from build123d import *

# Parameters (mm, degrees)
SKETCH1_R               = 5
BOSS_EXTRUDE1_DEPTH     = 50
CUT_EXTRUDE1_DEPTH      = 51.497524692
CUT_EXTRUDE1_DEPTH_BACK = 51.497524692
SKETCH2_W               = 0.5
SKETCH2_H               = 40
CHAMFER1_SIZE           = 3


with BuildPart() as part:
    # Sketch1 → Boss-Extrude1 (new body)
    with BuildSketch(Plane.XY):
        Circle(SKETCH1_R)
    extrude(amount=BOSS_EXTRUDE1_DEPTH)

    # Sketch2 → Cut-Extrude1 (cut, two sides: drawn at the far end of the back side and taken through both)
    with BuildSketch(Plane(origin=(0, 0, 0), x_dir=(1, 0, 0), z_dir=(0, 1, 0)).offset(-CUT_EXTRUDE1_DEPTH_BACK)):
        with Locations((0, -20)):
            Rectangle(SKETCH2_W, SKETCH2_H)
        Polygon((-5, -8), (-2, -8), (-2, -10), (-5, -11.732050808), align=None)
        Polygon((2, -10), (5, -11.732050808), (5, -8), (2, -8), align=None)
        Polygon((-5, -16), (-2, -16), (-2, -18), (-5, -19.732050808), align=None)
        Polygon((2, -16), (2, -18), (5, -19.732050808), (5, -16), align=None)
        Polygon((-5, -24), (-2, -24), (-2, -26), (-5, -27.732050808), align=None)
        Polygon((2, -24), (2, -26), (5, -27.732050808), (5, -24), align=None)
        Polygon((-5, -32), (-2, -32), (-2, -34), (-5, -35.732050808), align=None)
        Polygon((2, -32), (2, -34), (5, -35.732050808), (5, -32), align=None)
    extrude(amount=CUT_EXTRUDE1_DEPTH + CUT_EXTRUDE1_DEPTH_BACK, mode=Mode.SUBTRACT)

    # Chamfer1
    chamfer1_edges = [part.edges().sort_by_distance(p)[0] for p in [
        (-5, 0, 0),
        (3.622844187, -3.446012188, 0),
    ]]
    chamfer(chamfer1_edges, length=CHAMFER1_SIZE)

    # Cut-Extrude2 cone 1 section (through the dimple's axis) → Cut-Extrude2 (revolve, cut)
    with BuildSketch(Plane(origin=(0, 0, 50), x_dir=(0, -1, 0), z_dir=(1, 0, 0))):
        Polygon((0, 0), (4.5, 0), (0, 25.520768188), align=None)
    revolve(axis=Axis((0, 0, 50), (0, 0, -1)), mode=Mode.SUBTRACT)


solid = part.part
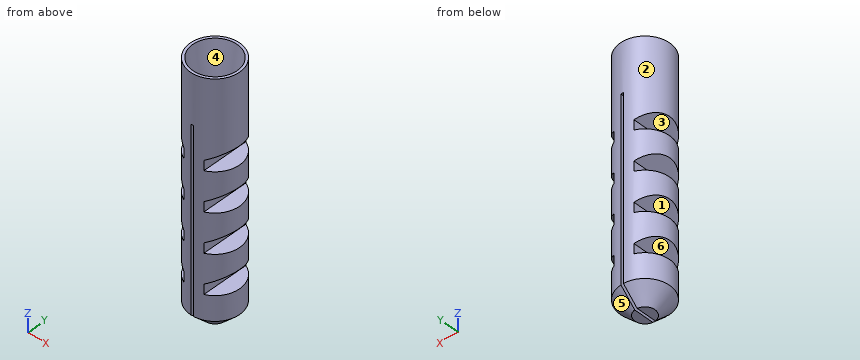
Verification items for the finished model (mm, model axes). Face numbers are marked on the shaded views. A direction names the side the tool comes from. Coordinates: 2 decimals unless noted, no trailing zeros. Order: outer loops, then holes, each group sorted by start corner. A loop starts at its lowest first (then second) coordinate and runs counter-clockwise, first axis right, second up. Notation, with made-up numbers: (63.5, -34) -> (90.5, -34) arc R28 ccw to (90.5, -2) -> close; hole circle Ø5 at (77, -24.75). An arc over 180 degrees is marked (long way). Use CSV: the item, a comma, the result in double quotes. Start each with the question number.
Q1. Draft check along Z on the marked faces 3, 4, 5 and 6. Enter one of: +Z half, -Z half, draft (parallel to the pull), parting line (faces both ways), or undercut.
Q2. Tool access check on the marked faces 1 and 2. Record the directions out of +Z, -Z, +X, -X, +Y, -Y that give a thin tool (end or side, any length) a straight path to the whole face; none if there is none.
Q3. Section check A-A, the plane z = 18.5. Record the cut outline in (x, y).
Q4. Thickness scan on line 1 along X through (y, z) = (0.25, 21.5); line 2 along X through (y, z) = (-1.25, 13); line 3 along Z through (x, y) = (-3.5, 3). Record the ranges inside material, lowest first.
Q5. Section check B-B, the plane x = -2.75. Give the number of separate pieces and of enclosed holes in the cut face, and give its area (3 significant figures).
Q6. Depth check by flat-ended pin: P1, Ø1, axis at y = -2, z = 9, coming from the -X side; P2, Ø1.6, axis at y = 1, z = 9, coming from the +X side; P3, Ø1.6, axis at y = 0.5, z = 17.5, coming from the -X side. Enter the tip coordinate at first touch or a pass-through.
Returned:
1,face 3,"undercut"
1,face 4,"+Z half"
1,face 5,"-Z half"
1,face 6,"undercut"
2,face 1,"-X, +Y, -Y"
2,face 2,"+Z, -Z"
3,outline,"(-2.87, -4.1) arc R5 ccw to (-0.25, -4.99) -> (-0.25, 4.99) arc R5 ccw to (-2.87, 4.1) -> close; (0.25, -4.99) arc R5 ccw to (2.87, -4.1) -> (2.87, 4.1) arc R5 ccw to (0.25, 4.99) -> close"
4,line 1,"x = -4.99 to -0.25, 0.25 to 4.99"
4,line 2,"x = -4.84 to -0.25, 0.25 to 4.84"
4,line 3,"z = 2.61 to 8, 10.87 to 16, 18.87 to 24, 26.87 to 32, 34.87 to 50"
5,separate pieces,"5"
5,enclosed holes,"0"
5,area,"278 mm^2"
6,P1,"stops at x = -2"
6,P2,"stops at x = 2"
6,P3,"stops at x = -2.52"
